CAD build for the part. Positions are in the model's coordinates, mm. A direction names the side the tool comes from. Round coordinates to 2 decimals unless told otherwise and drop trailing zeros. Order: outer loops, then holes, each group sorted by start corner. A loop starts at its lowest first (then second) coordinate and runs counter-clockwise, first axis right, second up. Notation, with made-up numbers: (2.5, 46.5) -> (48.5, 46.5) arc R10 cw to (48.5, 56.5) -> close; hole circle Ø1 at (76, -38). An arc over 180 degrees is marked (long way). Answer as CSV lines item,"result". Start each with the question number.
from build123d import *

# Parameters (mm, degrees)
SKETCH1_W           = 40
SKETCH1_H           = 44
SKETCH1_R           = 1.4
BOSS_EXTRUDE1_DEPTH = 3
SKETCH2_W           = 40
SKETCH2_H           = 15
BOSS_EXTRUDE2_DEPTH = 4.75
SKETCH3_W           = 40
SKETCH3_H           = 15
BOSS_EXTRUDE3_DEPTH = 4.75
CUT_EXTRUDE1_DEPTH  = 1.75
CUT_EXTRUDE2_REACH  = 53.75
SKETCH5_R           = 1.2
SKETCH5_R_2         = 2.75
CUT_EXTRUDE3_REACH  = 55.5
SKETCH6_R           = 2.38125
SKETCH7_R           = 1.190625
CUT_EXTRUDE4_DEPTH  = 16
CUT_EXTRUDE5_REACH  = 5
CUT_EXTRUDE6_REACH  = 55.5
FILLET1_R           = 1
CHAMFER1_SIZE       = 3.5
FILLET2_R           = 2.5


with BuildPart() as part:
    # Sketch1 → Boss-Extrude1 (new body)
    with BuildSketch(Plane(origin=(0, 0, 0), x_dir=(1, 0, 0), z_dir=(0, 1, 0))):
        Rectangle(SKETCH1_W, SKETCH1_H)
        with Locations((-14, 18)):
            Circle(SKETCH1_R, mode=Mode.SUBTRACT)
        with Locations((14, 18)):
            Circle(SKETCH1_R, mode=Mode.SUBTRACT)
        with Locations((-14, -18)):
            Circle(SKETCH1_R, mode=Mode.SUBTRACT)
        with Locations((14, -18)):
            Circle(SKETCH1_R, mode=Mode.SUBTRACT)
    extrude(amount=BOSS_EXTRUDE1_DEPTH)

    # Sketch2 → Boss-Extrude2 (add)
    with BuildSketch(Plane.XY.offset(22)):
        with Locations((0, 7.5)):
            Rectangle(SKETCH2_W, SKETCH2_H)
    extrude(amount=BOSS_EXTRUDE2_DEPTH)

    # Sketch3 → Boss-Extrude3 (add)
    with BuildSketch(Plane(origin=(0, 0, -22), x_dir=(-1, 0, 0), z_dir=(0, 0, -1))):
        with Locations((0, 7.5)):
            Rectangle(SKETCH3_W, SKETCH3_H)
    extrude(amount=BOSS_EXTRUDE3_DEPTH)

    # Sketch4 → Cut-Extrude1 (cut)
    with BuildSketch(Plane.XY.offset(26.75)):
        with BuildLine():
            Line((15.35, 12.98245603), (0.5, 14.474937186))
            ThreePointArc((0.5, 14.474937186), (0, 14.5), (-0.5, 14.474937186))
            Line((-0.5, 14.474937186), (-15.35, 12.98245603))
            ThreePointArc((-15.35, 12.98245603), (-18.5, 9.5), (-15.35, 6.01754397))
            Line((-15.35, 6.01754397), (-0.5, 4.525062814))
            ThreePointArc((-0.5, 4.525062814), (0, 4.5), (0.5, 4.525062814))
            Line((0.5, 4.525062814), (15.35, 6.01754397))
            ThreePointArc((15.35, 6.01754397), (18.5, 9.5), (15.35, 12.98245603))
        make_face()
    extrude(amount=-CUT_EXTRUDE1_DEPTH, mode=Mode.SUBTRACT)

    # Sketch5 → Cut-Extrude2 (cut, up to next)
    with BuildSketch(Plane.XY.offset(25), mode=Mode.PRIVATE) as cut_extrude2_sk1:
        with Locations((-15, 9.5)):
            Circle(SKETCH5_R)
    cut_extrude2_tool1 = extrude(cut_extrude2_sk1.sketch, amount=-CUT_EXTRUDE2_REACH, mode=Mode.PRIVATE) & part.part
    add(cut_extrude2_tool1.solids().sort_by_distance((-15, 9.5, 25))[0], mode=Mode.SUBTRACT)
    # Sketch5 → Cut-Extrude2 (cut, up to next)
    with BuildSketch(Plane.XY.offset(25), mode=Mode.PRIVATE) as cut_extrude2_sk2:
        with Locations((15, 9.5)):
            Circle(SKETCH5_R)
    cut_extrude2_tool2 = extrude(cut_extrude2_sk2.sketch, amount=-CUT_EXTRUDE2_REACH, mode=Mode.PRIVATE) & part.part
    add(cut_extrude2_tool2.solids().sort_by_distance((15, 9.5, 25))[0], mode=Mode.SUBTRACT)
    # Sketch5 → Cut-Extrude2 (cut, up to next)
    with BuildSketch(Plane.XY.offset(25), mode=Mode.PRIVATE) as cut_extrude2_sk3:
        with Locations((0, 9.5)):
            Circle(SKETCH5_R_2)
    cut_extrude2_tool3 = extrude(cut_extrude2_sk3.sketch, amount=-CUT_EXTRUDE2_REACH, mode=Mode.PRIVATE) & part.part
    add(cut_extrude2_tool3.solids().sort_by_distance((0, 9.5, 25))[0], mode=Mode.SUBTRACT)

    # Sketch6 → Cut-Extrude3 (cut, up to next)
    with BuildSketch(Plane(origin=(0, 0, -26.75), x_dir=(-1, 0, 0), z_dir=(0, 0, -1)), mode=Mode.PRIVATE) as cut_extrude3_sk1:
        with Locations((0, 9.5)):
            Circle(SKETCH6_R)
    cut_extrude3_tool1 = extrude(cut_extrude3_sk1.sketch, amount=-CUT_EXTRUDE3_REACH, mode=Mode.PRIVATE) & part.part
    add(cut_extrude3_tool1.solids().sort_by_distance((0, 9.5, -26.75))[0], mode=Mode.SUBTRACT)

    # Sketch7 → Cut-Extrude4 (cut, through all)
    with BuildSketch(Plane(origin=(0, 15, 0), x_dir=(1, 0, 0), z_dir=(0, 1, 0))):
        with Locations((0, 24.375)):
            Circle(SKETCH7_R)
    extrude(amount=-CUT_EXTRUDE4_DEPTH, mode=Mode.SUBTRACT)

    # Sketch8 → Cut-Extrude5 (cut, up to next)
    with BuildSketch(Plane(origin=(0, 3, 0), x_dir=(1, 0, 0), z_dir=(0, 1, 0)), mode=Mode.PRIVATE) as cut_extrude5_sk1:
        Polygon((-20, 18), (-17, 15), (-17, -15), (-20, -18), align=None)
    cut_extrude5_tool1 = extrude(cut_extrude5_sk1.sketch, amount=-CUT_EXTRUDE5_REACH, mode=Mode.PRIVATE) & part.part
    add(cut_extrude5_tool1.solids().sort_by_distance((-18.545455, 3, 0))[0], mode=Mode.SUBTRACT)
    # Sketch8 → Cut-Extrude5 (cut, up to next)
    with BuildSketch(Plane(origin=(0, 3, 0), x_dir=(1, 0, 0), z_dir=(0, 1, 0)), mode=Mode.PRIVATE) as cut_extrude5_sk2:
        Polygon((17, -15), (20, -18), (20, 18), (17, 15), align=None)
    cut_extrude5_tool2 = extrude(cut_extrude5_sk2.sketch, amount=-CUT_EXTRUDE5_REACH, mode=Mode.PRIVATE) & part.part
    add(cut_extrude5_tool2.solids().sort_by_distance((18.545455, 3, 0))[0], mode=Mode.SUBTRACT)

    # Sketch9 → Cut-Extrude6 (cut, up to next)
    with BuildSketch(Plane(origin=(0, 0, -26.75), x_dir=(-1, 0, 0), z_dir=(0, 0, -1)), mode=Mode.PRIVATE) as cut_extrude6_sk1:
        Polygon((-20, 15), (-4.995024308, 15), (-20, 3), align=None)
    cut_extrude6_tool1 = extrude(cut_extrude6_sk1.sketch, amount=-CUT_EXTRUDE6_REACH, mode=Mode.PRIVATE) & part.part
    add(cut_extrude6_tool1.solids().sort_by_distance((14.998341, 11, -26.75))[0], mode=Mode.SUBTRACT)
    # Sketch9 → Cut-Extrude6 (cut, up to next)
    with BuildSketch(Plane(origin=(0, 0, -26.75), x_dir=(-1, 0, 0), z_dir=(0, 0, -1)), mode=Mode.PRIVATE) as cut_extrude6_sk2:
        Polygon((20, 15), (5, 15), (20, 3), align=None)
    cut_extrude6_tool2 = extrude(cut_extrude6_sk2.sketch, amount=-CUT_EXTRUDE6_REACH, mode=Mode.PRIVATE) & part.part
    add(cut_extrude6_tool2.solids().sort_by_distance((-15, 11, -26.75))[0], mode=Mode.SUBTRACT)

    # Fillet1
    fillet1_edges = [part.edges().sort_by_distance(p)[0] for p in [
        (0, 3, -22),
        (0, 3, 22),
    ]]
    fillet(fillet1_edges, radius=FILLET1_R)

    # Chamfer1
    chamfer1_edges = [part.edges().sort_by_distance(p)[0] for p in [
        (-20, 15, 24.375),
        (20, 15, 24.375),
    ]]
    chamfer(chamfer1_edges, length=CHAMFER1_SIZE)

    # Fillet2
    fillet2_edges = [part.edges().sort_by_distance(p)[0] for p in [
        (4.995024308, 15, -24.375),
        (-5, 15, -24.375),
    ]]
    fillet(fillet2_edges, radius=FILLET2_R)


solid = part.part
Item 1: Mould opens along Y. For faces 4 (the flat face through (17, 2, 0)), 5 (the cylindrical face through (4.957, 14.855, -24.342)), 6 (the cylindrical face through (-14.446, 8.435, 23.521)), 7 (the flat face through (0, 0, 0)) say: released by +Y, released by -Y, zero draft, split by the parting line, or undercut.
Item 2: Tool access for faces 1 (the flat face through (-12.74, 8.81, -24.55)), 2 (the cylindrical face through (-0.358, 12.227, 23.521)), 3 (the flat face through (19, 2, -17)): list every direction of +Z, -Z, +X, -X, +Y, -Y with a clear straight run to the whole face (end or side of a thin tool).
Item 3: Pin check, flat tips, straight feed: pin 1 (8 mm diameter, centred on x = 15, z = -8.5, fed in from +Y); pin 2 (3.5 mm diameter, centred on x = 0, y = 9.5, fed in from +Z); pin 3 (5 mm diameter, centred on x = -6.5, y = 9, fed in from +Z); pin 4 (3.5 mm diameter, centred on y = 1, z = -5, fed in from -X). Stop position of each tip, or through.
Item 4: Band-saw the part on D-D, the plane y = 1. Give the cut face in (x, z) (3 decimals).
Item 5: Probe line 1 (Z direction, x = 14, y = 1.2); line 2 (Z direction, x = 0, y = 5); line 3 (X direction, y = 2.15, z = 18). List the from-to ranges inside material, lowest first.
Item 6: Band-saw the part on B-B, the plane y = 9.5. Give the cut face in (x, z) (3 decimals).
Item 7: Band-saw the part on C-C, the plane z = 16. Give the cut face in (x, y), and give its area (3 significant figures).
Item 8: Band-saw the part on A-A, the plane y = 13.75. Count the separate pieces of the cut face and the enclosed holes in it, and give its area (3 significant figures).
Values:
1,face 4,"zero draft"
1,face 5,"released by +Y"
1,face 6,"undercut"
1,face 7,"released by -Y"
2,face 1,"-Z, -X, +Y"
2,face 2,"+Z"
2,face 3,"+X, +Y, -Y"
3,pin 1,"y = 3"
3,pin 2,"through"
3,pin 3,"z = 25"
3,pin 4,"x = -17"
4,outline,"(-20, -26.75) -> (20, -26.75) -> (20, -18) -> (17, -15) -> (17, 15) -> (20, 18) -> (20, 26.75) -> (-20, 26.75) -> (-20, 18) -> (-17, 15) -> (-17, -15) -> (-20, -18) -> close; hole circle Ø2.8 at (-14, -18); hole circle Ø2.8 at (-14, 18); hole circle Ø2.381 at (0, -24.375); hole circle Ø2.8 at (14, -18); hole circle Ø2.8 at (14, 18)"
5,line 1,"-26.75 to -19.4, -16.6 to 16.6, 19.4 to 26.75"
5,line 2,"-26.75 to -25.57, -23.18 to -22, 22 to 25"
5,line 3,"-20 to -15.4, -12.6 to 12.6, 15.4 to 20"
6,outline,"(-20, 22) -> (-16.2, 22) -> (-16.2, 25) -> (-18.5, 25) -> (-18.5, 26.75) -> (-20, 26.75) -> close; (-13.8, 22) -> (-2.75, 22) -> (-2.75, 25) -> (-13.8, 25) -> close; (-11.875, -26.75) -> (-2.381, -26.75) -> (-2.381, -22) -> (-11.875, -22) -> close; (2.381, -26.75) -> (11.872, -26.75) -> (11.872, -22) -> (2.381, -22) -> close; (2.75, 22) -> (13.8, 22) -> (13.8, 25) -> (2.75, 25) -> close; (16.2, 22) -> (20, 22) -> (20, 26.75) -> (18.5, 26.75) -> (18.5, 25) -> (16.2, 25) -> close"
7,outline,"(-18, 0) -> (18, 0) -> (18, 3) -> (-18, 3) -> close"
7,area,"108 mm²"
8,separate pieces,"2"
8,enclosed holes,"1"
8,area,"199 mm²"
